from build123d import *

# Parameters (mm, degrees)
CHANFRO1_SIZE         = 0.7
FILETE1_R             = 0.5
ESBO_O5_R             = 1.4
CORTE_EXTRUS_O1_DEPTH = 3
CHANFRO3_SIZE         = 2.8
FILETE2_R             = 4


with BuildPart() as part:
    # Esboço1 → Revolução1 (revolve)
    with BuildSketch(Plane.XY):
        Polygon((0, 0), (0, 4.5), (35, 4.5), (35, 6), (63.5, 6), (63.5, 5), (66, 5), (66, 6), (76, 6), (76, 0), align=None)
    revolve(axis=Axis((76, 0, 0), (-1, 0, 0)))

    # Chanfro1
    chanfro1_edges = [part.edges().sort_by_distance(p)[0] for p in [
        (63.5, -6, 0),
        (35, -6, 0),
    ]]
    chamfer(chanfro1_edges, length=CHANFRO1_SIZE)

    # Filete1
    filete1_edges = [part.edges().sort_by_distance(p)[0] for p in [
        (76, -6, 0),
        (66, -6, 0),
    ]]
    fillet(filete1_edges, radius=FILETE1_R)

    # Esboço5 → Corte-extrusão1 (cut)
    with BuildSketch(Plane.ZY):
        with Locations(Location((0, 0, 0), (0, 0, 270))):
            Circle(ESBO_O5_R)
    extrude(amount=-CORTE_EXTRUS_O1_DEPTH, mode=Mode.SUBTRACT)

    # Chanfro3
    chanfro3_edges = [part.edges().sort_by_distance(p)[0] for p in [
        (0, 1.4, 0),
    ]]
    chamfer(chanfro3_edges, length=CHANFRO3_SIZE)

    # Filete2
    # the kernel refuses this fillet: 4 mm, written as the material it adds along each edge
    with BuildSketch(Plane(origin=(3, 0, 0), x_dir=(0, -1, 0), z_dir=(0, 0, -1))) as filete2_piece_1:
        with BuildLine():
            CenterArc((0.1510004, 4), FILETE2_R, 270, 18.194872339)
            Line((0.1510004, 0), (0.1510004, -0.08))
            Line((0.1510004, -0.08), (1.4, -0.08))
            Line((1.4, -0.08), (1.48, 0))
            ThreePointArc((1.48, 0), (1.48, 0.1), (1.424979992, 0.124))
            Line((1.424979992, 0.124), (1.4, 0.2))
        make_face()
    revolve(axis=Axis((3, 0, 0), (-1, 0, 0)))


solid = part.part
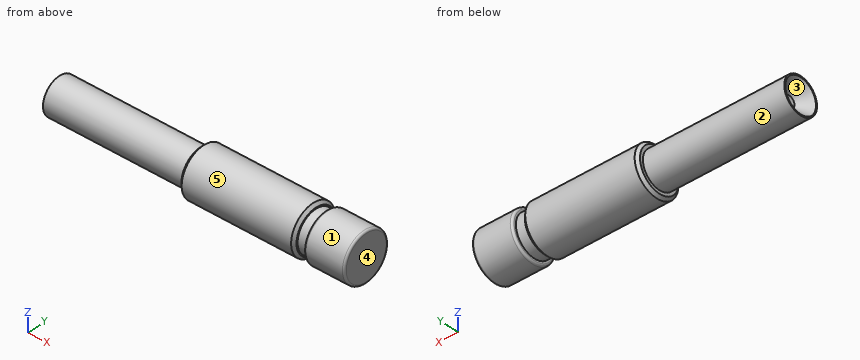
Read the model definition and answer for the solid it produces. Units are mm, in the model's axes. Face numbers are marked on the shaded views. A direction names the side the tool comes from. Round coordinates to 2 decimals unless told otherwise and drop trailing zeros. Order: outer loops, then holes, each group sorted by start corner. A loop starts at its lowest first (then second) coordinate and runs counter-clockwise, first axis right, second up.
1) The mould has two halves that part along Y. Classify the marked faces 3, 4 and 5: released by +Y, released by -Y, zero draft, split by the parting line, or undercut.
2) For the marked faces 1 and 2, determine the directions among +Z, -Z, +X, -X, +Y, -Y from which every point of the face is accessible in a straight line to the end or side of a thin tool.
3) A flat-ended cylindrical pin translates along its axis: pin 1 (2 mm diameter, centred on x = 21.5, y = 0, fed in from +Z). Find the tip coordinate at first contact, or state that the pin passes through.
4) The part is cut by section A-A on x = 24. Write down the section's boundary in (y, z), plus the area to 3 significant figures.
5) Straight lines are drawn through the part: L1, parallel to X at y = -3.5, z = 4; L2, parallel to X at y = 4.5, z = -3; L3, parallel to X at y = 1.75, z = -3. For each, find the intervals that lie inside material, in ascending order.
Resolved:
1. face 3: undercut
1. face 4: zero draft
1. face 5: split by the parting line
2. face 1: +X, -X
2. face 2: -X
3. pin 1: stops at z = 4.5
4. outline: circle Ø9 at (0, 0)
4. area: 63.6 mm2
5. L1: x = 35.02 to 63.48, 66 to 76
5. L2: x = 35.11 to 63.39, 66 to 76
5. L3: x = 0.73 to 76
